Design review of the part built by this model. Coordinates are the model's own, in mm. A direction names the side the tool comes from. Coordinates: 2 decimals unless noted, no trailing zeros. Write each loop counter-clockwise with the first axis right and the second up, starting at its lowest first coordinate (ties: lowest second). Pieces come first, ordered by that corner, then holes.
Q1. Take a section at B-B (z = -12). State how many separate pieces and enclosed holes the cut face has, and give its area (3 significant figures).
Q2. Insertion check: pin 1 (4 mm diameter, centred on y = 0.5, z = -8.5, fed in from +X); pin 2 (12 mm diameter, centred on y = -28.5, z = -6.5, fed in from -X); pin 3 (5 mm diameter, centred on x = 5, z = -24, fed in from +Y); pin 4 (10 mm diameter, centred on x = -10.5, y = -22.5, fed in from +Z). Each pin has a flat end and moves straight along its axis. Give the tip position at first contact, or say it passes through.
Q3. Take a section at C-C (z = -6). Give the boundary of the cut face in (x, y) (3 decimals), and give its area (3 significant figures).
Q4. Machinability: for faces 1 (the flat face through (-8, 8, -18)), 2 (the cylindrical face through (-2.11, -47.954, -22.93)), 3 (the cylindrical face through (-4.336, 19.524, 1.479)), which of the approach directions +Z, -Z, +X, -X, +Y, -Y give a long, thin tool a straight path to every point of the face, cutting with its end or side? Answer none if there is none.
Q5. For probe 1 along Y at (x, z) = (-14.5, -13); probe 2 along Y at (x, z) = (30.5, -17.5); probe 3 along Y at (x, z) = (0.5, -15.5), list the stretches that pass through material, from the lowest coordinate up.
Q6. Take a section at A-A (y = 0). Give the boundary of the cut face in (x, z), and give its area (3 significant figures).
Autodesk Inventor part; units mm, degrees
ref_plane "YZ Plane" through (0, 0, 0) normal (1, 0, 0) x (0, 1, 0)
ref_plane "XZ Plane" through (0, 0, 0) normal (0, 1, 0) x (-1, 0, 0)
ref_plane "XY Plane" through (0, 0, 0) normal (0, 0, 1) x (1, 0, 0)
sketch "Sketch1" plane through (0, 0, 0) normal (1, 0, 0) x (0, 1, 0)
  line L0 (0, 0) -> (0, -18)
  line L1 (37.5, 0) -> (48, -18)
  line L2 (37.5, 0) -> (0, 0)
  line L3 (46, -18.5407) -> (41.0179, -10)
  line L4 (41.0179, -10) -> (37.5, -10)
  line L5 (46, -18.5407) -> (46, -28)
  line L6 (46, -28) -> (48, -28)
  line L7 (48, -28) -> (48, -18)
  line L8 (0, -18) -> (37.5, -18)
  line L9 (37.5, -18) -> (37.5, -10)
  dimension "d0" = 18
  dimension "d6" = 75
  dimension "d7" = 96
  dimension "d9" = 10
  dimension "d10" = 10
  dimension "d11" = 2
  dimension "d12" = 2
revolve "Revolution1" add sketch "Sketch1" angle 360 about axis through (0, 0, 0) along (0, 0, -1)
sketch "Sketch2" plane through (0, 0, 0) normal (0, 0, 1) x (1, 0, 0)
  circle A0 centre (0, 0) radius 20
  point P0 (0, 0)
  dimension "d14" = 40
extrude "Extrusion1" add sketch "Sketch2" along normal blind 3
sketch "Sketch3" plane through (0, 0, -18) normal (0, 0, -1) x (-1, 0, 0)
  circle A0 centre (0, 0) radius 10
  point P0 (0, 0)
  dimension "d17" = 20
extrude "Extrusion2" cut sketch "Sketch3" against normal through all
sketch "Sketch4" plane through (0, 0, 0) normal (0, 0, 1) x (1, 0, 0)
  circle A0 centre (0, 27) radius 2.065
  point P0 (0, 0)
  dimension "d20" = 27
hole "Hole1" at (0, 27, 0) direction (0, 0, -1) diameter 5.5 end through all
thread "Thread2"
pattern_circular "Circular Pattern1" count 6 over 360 about axis through (0, 0, -9) along (0, 0, -1) of "Hole1"
properties part number "301-08" material "Titanium"
Response:
1. separate pieces: 2
1. enclosed holes: 8
1. area: 4,590 mm2
2. pin 1: stops at x = 43.62
2. pin 2: stops at x = -36.43
2. pin 3: stops at y = 47.93
2. pin 4: stops at z = 3
3. outline: circle Ø82 at (0, 0); hole circle Ø5.5 at (-23.383, -13.5); hole circle Ø5.5 at (-23.383, 13.5); hole circle Ø20 at (0, 0); hole circle Ø5.5 at (0, -27); hole circle Ø5.5 at (0, 27); hole circle Ø5.5 at (23.383, -13.5); hole circle Ø5.5 at (23.383, 13.5)
3. area: 4,820 mm2
4. face 1: -Z
4. face 2: +Z, -Z
4. face 3: +Z
5. probe 1: y = -42.69 to -40.23, -34.58 to 34.58, 40.23 to 42.69
5. probe 2: y = -36.69 to -33.62, -21.82 to 21.82, 33.62 to 36.69
5. probe 3: y = -46.54 to -44.22, -37.5 to -29.7, -24.3 to -9.99, 9.99 to 24.3, 29.7 to 37.5, 44.22 to 46.54
6. outline: (-48, -28) - (-46, -28) - (-46, -18.54) - (-41.02, -10) - (-37.5, -10) - (-37.5, -18) - (-10, -18) - (-10, 3) - (-20, 3) - (-20, 0) - (-37.5, 0) - (-48, -18) - close; (10, -18) - (37.5, -18) - (37.5, -10) - (41.02, -10) - (46, -18.54) - (46, -28) - (48, -28) - (48, -18) - (37.5, 0) - (20, 0) - (20, 3) - (10, 3) - close
6. area: 1,190 mm2
